from build123d import *

# Parameters (mm, degrees)
SKETCH_1_W          = 220
SKETCH_1_H          = 123.55
EXTRUDE_1_DEPTH     = 1.5
SKETCH_2_R          = 1.5
CUT_EXTRUDE_1_DEPTH = 10
SKETCH_3_W          = 35
SKETCH_3_H          = 10
SKETCH_3_W_2        = 25
SKETCH_3_H_2        = 15
CUT_EXTRUDE_2_DEPTH = 174.45613061
SKETCH_3_3_W        = 27
SKETCH_3_3_H        = 17
SKETCH_3_3_W_2      = 25
SKETCH_3_3_H_2      = 15
EXTRUDE_2_DEPTH     = 12
SKETCH_3_4_W        = 37
SKETCH_3_4_H        = 12
SKETCH_3_4_W_2      = 35
SKETCH_3_4_H_2      = 10
EXTRUDE_3_DEPTH     = 20
SKETCH_11_W         = 17
SKETCH_11_H         = 1
EXTRUDE_4_DEPTH     = 25
SKETCH_12_W         = 12
SKETCH_12_H         = 1
EXTRUDE_5_DEPTH     = 35


with BuildPart() as part:
    # 草图1 → 凸台-拉伸1 (new body)
    with BuildSketch(Plane(origin=(0, 0, 0), x_dir=(1, 0, 0), z_dir=(0, 1, 0))):
        with Locations((44.295012832, -17.457747405)):
            Rectangle(SKETCH_1_W, SKETCH_1_H)
    extrude(amount=EXTRUDE_1_DEPTH)

    # 草图2 → 切除-拉伸1 (cut)
    with BuildSketch(Plane(origin=(0, 1.5, 0), x_dir=(1, 0, 0), z_dir=(0, 1, 0))):
        with Locations(Location((149.295012832, -69.232747405, 0), (0, 0, 270))):
            Circle(SKETCH_2_R)
        with Locations(Location((149.295012832, -49.232747405, 0), (0, 0, 270))):
            Circle(SKETCH_2_R)
        with Locations(Location((44.295012832, -49.232747405, 0), (0, 0, 270))):
            Circle(SKETCH_2_R)
        with Locations(Location((44.295012832, -69.232747405, 0), (0, 0, 270))):
            Circle(SKETCH_2_R)
        with Locations(Location((44.295012832, 14.317252595, 0), (0, 0, 270))):
            Circle(SKETCH_2_R)
        with Locations(Location((44.295012832, 34.317252595, 0), (0, 0, 270))):
            Circle(SKETCH_2_R)
        with Locations(Location((149.295012832, 14.317252595, 0), (0, 0, 270))):
            Circle(SKETCH_2_R)
        with Locations(Location((149.295012832, 34.317252595, 0), (0, 0, 270))):
            Circle(SKETCH_2_R)
        with Locations(Location((-60.704987168, 34.317252595, 0), (0, 0, 270))):
            Circle(SKETCH_2_R)
        with Locations(Location((-60.704987168, 14.317252595, 0), (0, 0, 270))):
            Circle(SKETCH_2_R)
        with Locations(Location((-60.704987168, -49.232747405, 0), (0, 0, 270))):
            Circle(SKETCH_2_R)
        with Locations(Location((-60.704987168, -69.232747405, 0), (0, 0, 270))):
            Circle(SKETCH_2_R)
        with Locations(Location((-60.704987168, -29.232747405, 0), (0, 0, 270))):
            Circle(SKETCH_2_R)
        with Locations(Location((-60.704987168, -5.682747405, 0), (0, 0, 270))):
            Circle(SKETCH_2_R)
        with Locations(Location((44.295012832, -5.682747405, 0), (0, 0, 270))):
            Circle(SKETCH_2_R)
        with Locations(Location((44.295012832, -29.232747405, 0), (0, 0, 270))):
            Circle(SKETCH_2_R)
        with Locations(Location((149.295012832, -5.682747405, 0), (0, 0, 270))):
            Circle(SKETCH_2_R)
        with Locations(Location((149.295012832, -29.232747405, 0), (0, 0, 270))):
            Circle(SKETCH_2_R)
    extrude(amount=-CUT_EXTRUDE_1_DEPTH, mode=Mode.SUBTRACT)

    # 草图3 → 切除-拉伸2 (cut, through all)
    with BuildSketch(Plane(origin=(0, 1.5, 0), x_dir=(1, 0, 0), z_dir=(0, 1, 0))):
        with Locations((-8.204987168, -58.232747405)):
            Rectangle(SKETCH_3_W, SKETCH_3_H)
        with Locations((-8.204987168, -21.732747405)):
            Rectangle(SKETCH_3_W_2, SKETCH_3_H_2)
    extrude(amount=-CUT_EXTRUDE_2_DEPTH, mode=Mode.SUBTRACT)

    # 草图3<3> → 凸台-拉伸2 (add)
    with BuildSketch(Plane(origin=(0, 1.5, 0), x_dir=(1, 0, 0), z_dir=(0, 1, 0))):
        with Locations((-8.204987168, -21.732747405)):
            Rectangle(SKETCH_3_3_W, SKETCH_3_3_H)
        with Locations((-8.204987168, -21.732747405)):
            Rectangle(SKETCH_3_3_W_2, SKETCH_3_3_H_2, mode=Mode.SUBTRACT)
    extrude(amount=EXTRUDE_2_DEPTH)

    # 草图3<4> → 凸台-拉伸3 (add)
    with BuildSketch(Plane(origin=(0, 1.5, 0), x_dir=(1, 0, 0), z_dir=(0, 1, 0))):
        with Locations((-8.204987168, -58.232747405)):
            Rectangle(SKETCH_3_4_W, SKETCH_3_4_H)
        with Locations((-8.204987168, -58.232747405)):
            Rectangle(SKETCH_3_4_W_2, SKETCH_3_4_H_2, mode=Mode.SUBTRACT)
    extrude(amount=EXTRUDE_3_DEPTH)

    # 草图11 → 凸台-拉伸4 (add)
    with BuildSketch(Plane(origin=(-20.704987168, 0, 0), x_dir=(0, 0, -1), z_dir=(1, 0, 0))):
        with Locations((-21.732747405, 13)):
            Rectangle(SKETCH_11_W, SKETCH_11_H)
    extrude(amount=EXTRUDE_4_DEPTH)

    # 草图12 → 凸台-拉伸5 (add)
    with BuildSketch(Plane(origin=(-25.704987168, 0, 0), x_dir=(0, 0, -1), z_dir=(1, 0, 0))):
        with Locations((-58.232747405, 21)):
            Rectangle(SKETCH_12_W, SKETCH_12_H)
    extrude(amount=EXTRUDE_5_DEPTH)


solid = part.part
Can you work these out from the model? Positions are in its coordinate system, mm. A direction names the side the tool comes from. Give positions to 0.01 mm unless a question says otherwise; leave off trailing zeros. Loops run counter-clockwise (first coordinate to the right, second up) from the corner with the lowest first, then second, coordinate; pieces in that order, holes last. Notation, with made-up numbers: (-19.75, -28) - (3.25, -28) arc R26 ccw to (3.25, 3) - close; hole circle Ø1 at (66.5, 49.5). An arc over 180 degrees is marked (long way). Return JSON: item names as keys, results as strings.
1. If I drill on line 1 (Z direction, x = -10.5, y = 9.75); line 2 (X direction, y = 16, z = 54); line 3 (Z direction, x = -4, y = 16.25), over which ranges is the centre line in solid material (lowest first)?
Output values:
{"line 1": "z = 13.23 to 14.23, 29.23 to 30.23, 52.23 to 53.23, 63.23 to 64.23", "line 2": "x = -26.7 to -25.7, 9.3 to 10.3", "line 3": "z = 52.23 to 53.23, 63.23 to 64.23"}
2. We'd pull the mould along Z, two halves only. Please class faces 6 (the face through (-8, 11, 64.233)), 7 (the face through (-26.705, 11, 58)), 8 (the face through (-25.705, 10, 58)), 9 (the face through (-8, 12.5, 22)): +Z half, -Z half, draft (parallel to the pull), parting line (faces both ways), or undercut.
Output values:
{"face 6": "+Z half", "face 7": "draft", "face 8": "undercut", "face 9": "undercut"}
3. I'm going to push flat-ended pins straight in: pin 1 Ø2.5 at (x, z) = (-60.7, -34.32) entering from +Y; pin 2 Ø5 at (x, z) = (44.3, -34.32) entering from +Y; pin 3 Ø10 at (x, y) = (-12.5, 11.5) entering from +Z; pin 4 Ø8 at (y, z) = (7.5, 60) entering from +X (3 decimals). Where does each tip first touch, or does it pass through?
Output values:
{"pin 1": "passes through", "pin 2": "stops at y = 1.5", "pin 3": "stops at z = 64.23", "pin 4": "stops at x = 10.295"}
4. I want a section at A-A on y = 9.5. Please give me the cut outline in (x, z), and give its area (3 significant figures).
Output values:
{"outline": "(-26.7, 52.23) - (10.3, 52.23) - (10.3, 64.23) - (-26.7, 64.23) - close; (-21.7, 13.23) - (5.3, 13.23) - (5.3, 30.23) - (-21.7, 30.23) - close; hole (-25.7, 53.23) - (9.3, 53.23) - (9.3, 63.23) - (-25.7, 63.23) - close; hole (-20.7, 14.23) - (4.3, 14.23) - (4.3, 29.23) - (-20.7, 29.23) - close", "area": "178 mm²"}
5. I want a section at D-D on x = 85.5. Please give me the cut outline in (y, z).
Output values:
{"outline": "(0, -44.32) - (1.5, -44.32) - (1.5, 79.23) - (0, 79.23) - close"}
6. I want a section at C-C on z = 20. Please give me the cut outline in (x, y).
Output values:
{"outline": "(-65.7, 0) - (-20.7, 0) - (-20.7, 12.5) - (4.3, 12.5) - (4.3, 0) - (154.3, 0) - (154.3, 1.5) - (5.3, 1.5) - (5.3, 13.5) - (-21.7, 13.5) - (-21.7, 1.5) - (-65.7, 1.5) - close"}
7. For faces 1 (the face through (-8, 7, 13.233)), 2 (the face through (-8, 7, 30.233)), 3 (the face through (10.295, 11, 58)), 4 (the face through (-21.705, 7, 22)), 5 (the face through (9.295, 10, 58)), which set-ups out of +Z, -Z, +X, -X, +Y, -Y let a thin tool reach every point of the face, with its end or its side?
Output values:
{"face 1": "-Z, +X, -X, +Y", "face 2": "+X, -X, +Y", "face 3": "+Z, -Z, +X, +Y", "face 4": "-Z, -X, +Y", "face 5": "-Y"}
8. I want a section at B-B on x = 1.5. Please give me the cut outline in (y, z), and give its area (3 significant figures).
Output values:
{"outline": "(0, -44.32) - (1.5, -44.32) - (1.5, 13.23) - (13.5, 13.23) - (13.5, 30.23) - (1.5, 30.23) - (1.5, 52.23) - (21.5, 52.23) - (21.5, 64.23) - (1.5, 64.23) - (1.5, 79.23) - (0, 79.23) - (0, 63.23) - (20.5, 63.23) - (20.5, 53.23) - (0, 53.23) - (0, 29.23) - (12.5, 29.23) - (12.5, 14.23) - (0, 14.23) - close", "area": "237 mm²"}
